from build123d import *

# Parameters (mm, degrees)
SKETCH1_W           = 210
SKETCH1_H           = 6
BOSS_EXTRUDE1_DEPTH = 15
SKETCH2_RX          = 12.084795348
SKETCH2_RY          = 9.25941939
BOSS_EXTRUDE2_DEPTH = 15
SKETCH3_R           = 3.15
CUT_EXTRUDE1_DEPTH  = 15
BOSS_EXTRUDE3_DEPTH = 15
SKETCH5_R           = 5.15
CUT_EXTRUDE2_DEPTH  = 2
SKETCH6_R           = 5.15
CUT_EXTRUDE3_DEPTH  = 2


with BuildPart() as part:
    # Sketch1 → Boss-Extrude1 (new body)
    with BuildSketch(Plane.XY):
        with Locations((19.744707347, 18.183063512)):
            Rectangle(SKETCH1_W, SKETCH1_H)
    extrude(amount=BOSS_EXTRUDE1_DEPTH)

    # Sketch2 → Boss-Extrude2 (add)
    with BuildSketch(Plane.XY.offset(15)):
        with Locations((19.744707347, 18.183063512)):
            Ellipse(SKETCH2_RX, SKETCH2_RY)
    extrude(amount=-BOSS_EXTRUDE2_DEPTH)

    # Sketch3 → Cut-Extrude1 (cut)
    with BuildSketch(Plane.XY.offset(15)):
        with Locations((19.744707347, 18.183063512)):
            Circle(SKETCH3_R)
    extrude(amount=-CUT_EXTRUDE1_DEPTH, mode=Mode.SUBTRACT)

    # Sketch4 → Boss-Extrude3 (add)
    with BuildSketch(Plane.XY.offset(15)):
        with BuildLine():
            Line((17.144707347, 19.961405436), (17.144707347, 16.404721587))
            ThreePointArc((17.144707347, 16.404721587), (16.583900133, 18.183063512), (17.144707347, 19.961405436))
        make_face()
    extrude(amount=-BOSS_EXTRUDE3_DEPTH)

    # Sketch5 → Cut-Extrude2 (cut)
    with BuildSketch(Plane.XZ.offset(-15.183063512)):
        with Locations((-42.255292653, 7.5)):
            Circle(SKETCH5_R)
        with Locations((-66.755292653, 7.5)):
            Circle(SKETCH5_R)
    extrude(amount=-CUT_EXTRUDE2_DEPTH, mode=Mode.SUBTRACT)

    # Sketch6 → Cut-Extrude3 (cut)
    with BuildSketch(Plane(origin=(0, 21.183063512, 0), x_dir=(1, 0, 0), z_dir=(0, 1, 0))):
        with Locations((81.744707347, -7.5)):
            Circle(SKETCH6_R)
        with Locations((106.244707347, -7.5)):
            Circle(SKETCH6_R)
    extrude(amount=-CUT_EXTRUDE3_DEPTH, mode=Mode.SUBTRACT)


solid = part.part
Work out the finished part from the listing and answer in its coordinate system (mm). A direction names the side the tool comes from. Coordinates: 2 decimals unless noted, no trailing zeros. Loops run counter-clockwise (first coordinate to the right, second up) from the corner with the lowest first, then second, coordinate; pieces in that order, holes last. Notation, with made-up numbers: (-29.75, 57) -> (-25.75, 57) arc R33 ccw to (-25.75, 92) -> close; hole circle Ø9 at (48, -24). An arc over 180 degrees is marked (long way). Write each question's results on one line, items separated by ' | '. Start each with the question number.
1) The mould has two halves that part along Z. Classify faces 1 (the flat face through (21, 22, 0)), 2 (the cylindrical face through (-43.372, 16.169, 2.472)), 3 (the cylindrical face through (105.128, 20.197, 12.528)), 4 (the flat face through (-85.255, 18, 7)): pulls with the +Z half, pulls with the -Z half, needs draft (parallel to the pull), parting line crosses it, or undercut.
2) Consider line 1 along X through (y, z) = (15.75, 11); line 2 along X through (y, z) = (15.75, 12.25); line 3 along Y through (x, z) = (-58, 12.5). Determine where each line is inside the solid, lowest interval first.
3) Flat-ended cylindrical pins translate along their axes: P1, Ø5, axis at y = 15, z = 11.5, coming from the +X side; P2, Ø3, axis at x = -43, z = 6, coming from the -Y side; P3, Ø6, axis at x = -60.5, z = 4, coming from the -Y side; P4, Ø8, axis at x = 107, z = 6, coming from the +Y side. Find the tip coordinate at first contact, or state that the pin passes through.
4) Find section B-B on x = -13.5. Determine the outline of the cut face in (y, z).
5) Find section A-A on x = 103.5. Determine the outline of the cut face in (y, z), then the cut area to 3 significant figures.
6) For faces 5 (the flat face through (-67, 17.183, 8)), 6 (the flat face through (77, 15.183, 7)), 7 (the flat face through (17.145, 18, 8)), determine the directions among +Z, -Z, +X, -X, +Y, -Y from which every point of the face is accessible in a straight line to the end or side of a thin tool.
Response values:
1) face 1: pulls with the -Z half | face 2: undercut | face 3: undercut | face 4: needs draft
2) line 1: x = -85.26 to -70.53, -62.98 to -46.03, -38.48 to 17.74, 21.75 to 124.74 | line 2: x = -85.26 to -68.75, -64.77 to -44.25, -40.27 to 17.74, 21.75 to 124.74 | line 3: y = 15.18 to 21.18
3) P1: stops at x = 124.74 | P2: stops at y = 17.18 | P3: stops at y = 15.18 | P4: stops at y = 21.18
4) outline: (15.18, 0) -> (21.18, 0) -> (21.18, 15) -> (15.18, 15) -> close
5) outline: (15.18, 0) -> (21.18, 0) -> (21.18, 3.14) -> (19.18, 3.14) -> (19.18, 11.86) -> (21.18, 11.86) -> (21.18, 15) -> (15.18, 15) -> close | area: 72.6 mm^2
6) face 5: -Y | face 6: +Z, -Z, +X, -Y | face 7: +Z, -Z
